Can you work these out from the model? Positions are in its coordinate system, mm. A direction names the side the tool comes from. Give positions to 0.01 mm unless a question says otherwise; leave off trailing zeros. Loops run counter-clockwise (first coordinate to the right, second up) from the corner with the lowest first, then second, coordinate; pieces in that order, holes last. Notation, with made-up numbers: (17, 64.5) -> (56, 64.5) arc R25 cw to (56, 81.5) -> close; hole circle Ø5 at (11.5, -23). An arc over 180 degrees is marked (long way). Use CSV: the item, a comma, the result in double quotes.
from build123d import *

# Parameters (mm, degrees)
F1_DEPTH = 25.4


with BuildPart() as f1:
    # F0 (on Top) → F1 (new body)
    with BuildSketch(Plane.XY):
        with BuildLine():
            Line((0, 10.867205), (0, 73.025))
            Line((0, 73.025), (21.59, 73.025))
            Line((21.59, 73.025), (21.59, 51.435))
            Line((21.59, 51.435), (19.05, 51.435))
            Line((19.05, 51.435), (21.59, 46.355))
            Line((21.59, 46.355), (25.4, 46.355))
            Line((25.4, 46.355), (25.4, 76.835))
            Line((25.4, 76.835), (-2.974549, 76.835))
            ThreePointArc((-2.974549, 76.835), (-4.534456, 76.589572), (-5.943638, 75.877004))
            Line((-5.943638, 75.877004), (-51.515202, 43.051709))
            ThreePointArc((-51.515202, 43.051709), (-53.559832, 39.747649), (-52.671324, 35.965073))
            ThreePointArc((-52.671324, 35.965073), (-62.067004, 14.925134), (-75.741455, 33.471487))
            ThreePointArc((-75.741455, 33.471487), (-77.065813, 36.81054), (-80.404866, 35.486182))
            ThreePointArc((-80.404866, 35.486182), (-80.268512, 20.571789), (-69.132008, 10.650296))
            Line((-69.132008, 10.650296), (0, -11.557))
            Line((0, -11.557), (0, -3.937))
            Line((0, -3.937), (7.62, -3.937))
            Line((7.62, -3.937), (7.62, 1.143))
            Line((7.62, 1.143), (1.487898, 7.275102))
            ThreePointArc((1.487898, 7.275102), (0.386692, 8.923173), (0, 10.867205))
        make_face()
        with BuildLine():
            ThreePointArc((-14.184544, 57.419772), (-11.542231, 57.61956), (-10.16, 55.358771))
            Line((-10.16, 55.358771), (-10.16, 5.86179))
            ThreePointArc((-10.16, 5.86179), (-11.203595, 3.809384), (-13.476829, 3.443498))
            Line((-13.476829, 3.443498), (-41.841771, 12.555177))
            ThreePointArc((-41.841771, 12.555177), (-43.438593, 14.069376), (-43.253729, 16.262196))
            ThreePointArc((-43.253729, 16.262196), (-40.129208, 25.770222), (-41.245404, 35.71604))
            ThreePointArc((-41.245404, 35.71604), (-41.258358, 37.305502), (-40.324046, 38.591434))
            Line((-40.324046, 38.591434), (-14.184544, 57.419772))
        make_face(mode=Mode.SUBTRACT)
    extrude(amount=F1_DEPTH)


solid = f1.part
(1) Which directions (+Z, -Z, +X, -X, +Y, -Y) give clear straight access to the entire face, cutting with the end or side of a thin tool? Please do faces 1 (the face through (-28.4, 59.7, 12.5)), 2 (the face through (-9, 33, 25.4)), 3 (the face through (21.59, 62, 13)), 4 (the face through (0.397, 8.897, 12.522)), 5 (the face through (20.302, 48.931, 12.522)).
Answer sheet:
face 1,"+Z, -Z, -X, +Y"
face 2,"+Z, +X, -X, +Y, -Y"
face 3,"+Z, -Z"
face 4,"+Z, -Z, +X"
face 5,"+Z, -Z, -Y"
(2) If we section it at D-D, the plane y = 8.5: Write out the boundary of the cut face in (x, z), then the cut area to 3 significant figures.
Answer sheet:
outline,"(-62.44, 0) -> (-29.22, 0) -> (-29.22, 25.4) -> (-62.44, 25.4) -> close; (-10.16, 0) -> (0.59, 0) -> (0.59, 25.4) -> (-10.16, 25.4) -> close"
area,"1,120 mm2"
(3) If we section it at A-A, the plane y = 54: Write out the boundary of the cut face in (x, z), then the cut area to 3 significant figures.
Answer sheet:
outline,"(-36.32, 0) -> (-18.93, 0) -> (-18.93, 25.4) -> (-36.32, 25.4) -> close; (-10.16, 0) -> (0, 0) -> (0, 25.4) -> (-10.16, 25.4) -> close; (21.59, 0) -> (25.4, 0) -> (25.4, 25.4) -> (21.59, 25.4) -> close"
area,"796 mm2"
(4) We'd pull the mould along X, two halves only. Please class faces 6 (the face through (-11.58, 57.64, 12.52)), 7 (the face through (4, -3.937, 13)), 8 (the face through (7.62, -1, 13)): released by +X, released by -X, zero draft, split by the parting line, or undercut.
Answer sheet:
face 6,"undercut"
face 7,"zero draft"
face 8,"released by +X"
(5) If I drill on L1, parallel to X at y = 30.5, z = 7; L2, parallel to X at y = 57, z = 23.75; L3, parallel to Y at x = 10, z = 21 (3 decimals), over which ranges is the centre line in solid material (lowest first)? Write a range as from..to.
Answer sheet:
L1,"x = -81.77..-76.63, -50.37..-40.12, -10.16..0"
L2,"x = -32.15..-14.77, -10.76..0, 21.59..25.4"
L3,"y = 73.025..76.835"
(6) Will these pins go through, and if not, where does the flat tip stop? pin 1 Ø4 at (y, z) = (5.5, 7) entering from +X; pin 2 Ø1.9 at (x, z) = (23.5, 14) entering from -Y (3 decimals); pin 3 Ø6 at (y, z) = (39, 12) entering from -X.
Answer sheet:
pin 1,"stops at x = 5.26"
pin 2,"stops at y = 46.355"
pin 3,"stops at x = -80.11"
(7) If we section it at B-B, the plane x = 4: Write out the boundary of the cut face in (y, z) (3 decimals), then the cut area to 3 significant figures.
Answer sheet:
outline,"(-3.937, 0) -> (4.763, 0) -> (4.763, 25.4) -> (-3.937, 25.4) -> close; (73.025, 0) -> (76.835, 0) -> (76.835, 25.4) -> (73.025, 25.4) -> close"
area,"318 mm2"
